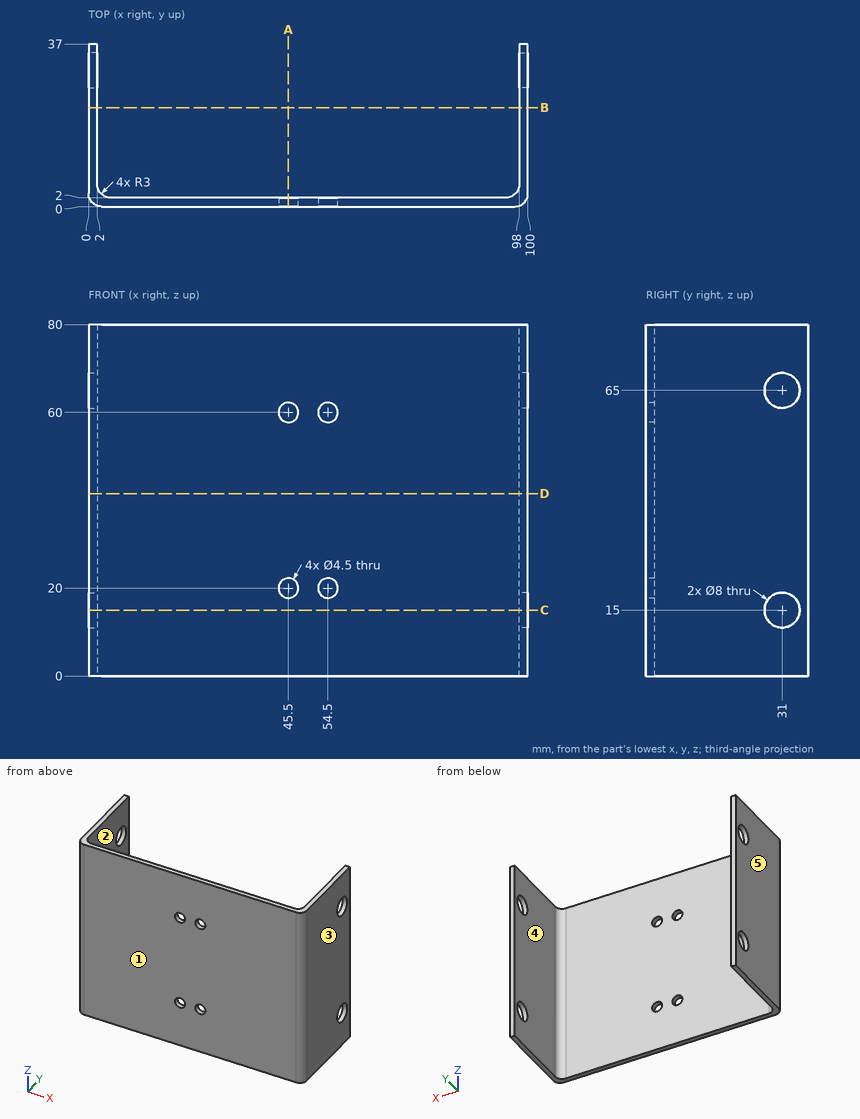
Design review of the part shown in the three views and the two pictorial views. Dimensions are in mm from the part's minimum x, y and z. A direction names the side the tool comes from. Coordinates: 2 decimals unless noted, no trailing zeros. Loops run counter-clockwise (first coordinate to the right, second up) from the corner with the lowest first, then second, coordinate; pieces in that order, holes last. Notation, with made-up numbers: M 78.5,49.5 L 97.5,49.5 A12 cw 97.5,53.5 Z; hole C 29,26 d3. An arc over 180 degrees is marked long. Put each result on its own line as item: value. Start each with the question number.
Q1. Add section A-A (x = 45.5). Write out the cut boundary in (y, z), and give its area (3 significant figures).
Q2. Add section B-B (y = 22.5). Write out the cut boundary in (x, z).
Q3. Wall thickness on line 1 (Z direction, x = 45.5, y = 1.3); line 2 (X direction, y = 18.5, z = 16.5); line 3 (Y direction, x = 84, z = 65): over which ranges is each line inside the solid? List them lowest first.
Q4. Add section D-D (z = 41.5). Write out the cut boundary in (x, y), and give its area (3 significant figures).
Q5. For the marked faces 1 and 2, list the 3-axis set-ups (+Z, -Z, +X, -X, +Y, -Y) from which the entire face can be reached by the end or side of a thin tool; tool diameter is ignored.
Q6. Add section C-C (z = 15). Write out the cut boundary in (x, y).
Q7. Clearance check with flat-ended pins moving along their axes: pin 1 (5 mm diameter, centred on y = 31, z = 15, fed in from -X); pin 2 (12 mm diameter, centred on x = 78, z = 41.5, fed in from +Y). State where each tip first meets the part, or that it passes through.
Q8. The part is to be moulded in two halves that separate along X. For the marked faces 3, 4 and 5, say which applies: +X half, -X half, draft (parallel to the pull), parting line (faces both ways), or undercut.
Answers:
1. outline: M 0,0 L 2,0 L 2,17.75 L 0,17.75 Z; M 0,22.25 L 2,22.25 L 2,57.75 L 0,57.75 Z; M 0,62.25 L 2,62.25 L 2,80 L 0,80 Z
1. area: 142 mm^2
2. outline: M 0,0 L 2,0 L 2,80 L 0,80 Z; M 98,0 L 100,0 L 100,80 L 98,80 Z
3. line 1: z = 0 to 17.75, 22.25 to 57.75, 62.25 to 80
3. line 2: x = 0 to 2, 98 to 100
3. line 3: y = 0 to 2
4. outline: M 0,3 A3 ccw 3,0 L 97,0 A3 ccw 100,3 L 100,37 L 98,37 L 98,5 A3 cw 95,2 L 5,2 A3 cw 2,5 L 2,37 L 0,37 Z
4. area: 340 mm^2
5. face 1: +Z, -Z, +X, -X, -Y
5. face 2: +Z, -Z, +Y
6. outline: M 0,3 A3 ccw 3,0 L 97,0 A3 ccw 100,3 L 100,27 L 98,27 L 98,5 A3 cw 95,2 L 5,2 A3 cw 2,5 L 2,27 L 0,27 Z; M 0,35 L 2,35 L 2,37 L 0,37 Z; M 98,35 L 100,35 L 100,37 L 98,37 Z
7. pin 1: passes through
7. pin 2: stops at y = 2
8. face 3: +X half
8. face 4: undercut
8. face 5: -X half
